Build history of the part. All positions in model axes, mm. A direction names the side the tool comes from. Round coordinates to 2 decimals unless told otherwise and drop trailing zeros. Loops run counter-clockwise (first coordinate to the right, second up) from the corner with the lowest first, then second, coordinate; pieces in that order, holes last. Notation, with made-up numbers: (39, -12.5) -> (86, -12.5) arc R14 cw to (86, 5.5) -> close; hole circle Ø2 at (1.25, 70). An arc over 180 degrees is marked (long way). Put each result on its own line as item: value. Start each with the question number.
Item 1: Tool access for faces 4 (the cylindrical face through (-33.345, 0.986, -28.568)), 5 (the cylindrical face through (36.649, 2.991, 26.096)), 6 (the cylindrical face through (-17.3, 3, 25.3)), 7 (the cylindrical face through (-30.1, 2.9, 21)): list every direction of +Z, -Z, +X, -X, +Y, -Y with a clear straight run to the whole face (end or side of a thin tool).
Item 2: Flat gauge pins, fed straight in: pin 1 Ø1.5 at (x, y) = (-6, 5) entering from -Z; pin 2 Ø3 at (x, y) = (-2.5, 2.5) entering from +Z; pin 3 Ø3 at (y, z) = (3.5, 22.5) entering from +X. Where does each tip first touch, or does it go through?
Item 3: Cut at B-B, the plane x = -1. List the corners of the cut face in (y, z).
Item 4: Pull direction X, two halves, no side cores. Call faces 1 (the flat face through (1, 0, -6)), 2 (the flat face through (29.39, 2.91, 31.54)), 3 (the cylindrical face through (-20.796, 2.909, 36.172)): +X half, -X half, draft (parallel to the pull), parting line (faces both ways), or undercut.
Item 5: Cut at A-A, the plane y = 4.7. Count the separate pieces of the cut face and the enclosed holes in it, plus the area to 3 significant figures.
Item 6: Drill centre lines: probe 1 along X at (y, z) = (2.8, -14.5); probe 2 along X at (y, z) = (0.3, 3.5); probe 3 along X at (y, z) = (0.85, -35). Where is each one in solid material? Low to high. Write a range as [from, to].
Item 7: Cut at D-D, the plane z = 15. List the corners of the cut face in (x, y), plus the area to 3 significant figures.
Item 8: Cut at C-C, the plane x = -46.5. List the corners of the cut face in (y, z).
```python
from build123d import *

# Parameters (mm, degrees)
RESSALTO_EXTRUS_O1_DEPTH = 5.9
FILETE1_R                = 8
FILETE2_R                = 3
ESBO_O2_R                = 1.5
CORTE_EXTRUS_O2_DEPTH    = 2
ESBO_O4_R                = 1.5
ESBO_O4_R_2              = 1.9
CORTE_EXTRUS_O3_DEPTH    = 78.327505241


with BuildPart() as part:
    # Esboço1 → Ressalto-extrusão1 (new body)
    with BuildSketch(Plane(origin=(0, 0, 0), x_dir=(1, 0, 0), z_dir=(0, 1, 0))):
        with BuildLine():
            Line((19.75, -23.063762314), (-19.75, -23.063762314))
            Line((-19.75, -23.063762314), (-19.75, -34.413762314))
            ThreePointArc((-19.75, -34.413762314), (-20.823151937, -36.186035619), (-22.890952667, -36.056390395))
            Line((-22.890952667, -36.056390395), (-37, -26.256390395))
            Line((-37, -26.256390395), (-37, -18.556390395))
            ThreePointArc((-37, -18.556390395), (-37.501443682, -9.224461006), (-39, 0))
            Line((-39, 0), (-60, 39.799497484))
            ThreePointArc((-60, 39.799497484), (-59.849748252, 45.058892271), (-55.268281966, 47.646164151))
            Line((-55.268281966, 47.646164151), (-49.818281966, 47.646164151))
            Line((-49.818281966, 47.646164151), (-16.15, 25.136237686))
            Line((-16.15, 25.136237686), (16.15, 25.136237686))
            Line((16.15, 25.136237686), (49.818281966, 47.646164151))
            Line((49.818281966, 47.646164151), (55.268281966, 47.646164151))
            ThreePointArc((55.268281966, 47.646164151), (59.849748252, 45.058892271), (60, 39.799497484))
            Line((60, 39.799497484), (39, 0))
            ThreePointArc((39, 0), (37.501443682, -9.224461006), (37, -18.556390395))
            Line((37, -18.556390395), (37, -26.256390395))
            Line((37, -26.256390395), (22.890952667, -36.056390395))
            ThreePointArc((22.890952667, -36.056390395), (20.823151937, -36.186035619), (19.75, -34.413762314))
            Line((19.75, -34.413762314), (19.75, -23.063762314))
        make_face()
    extrude(amount=RESSALTO_EXTRUS_O1_DEPTH)

    # Filete1
    filete1_edges = [part.edges().sort_by_distance(p)[0] for p in [
        (19.75, 2.95, 23.063762314),
        (-19.75, 2.95, 23.063762314),
    ]]
    fillet(filete1_edges, radius=FILETE1_R)

    # Filete2
    filete2_edges = [part.edges().sort_by_distance(p)[0] for p in [
        (-37, 2.95, 26.256390395),
        (-39, 2.95, 0),
        (-49.818281966, 2.95, -47.646164151),
        (-16.15, 2.95, -25.136237686),
        (16.15, 2.95, -25.136237686),
        (49.818281966, 2.95, -47.646164151),
        (39, 2.95, 0),
        (37, 2.95, 26.256390395),
    ]]
    fillet(filete2_edges, radius=FILETE2_R)

    # Esboço2 → Corte-extrusão2 (cut)
    # profile 1 of 2: a face of its own
    with BuildSketch(Plane.XZ):
        with BuildLine():
            Line((-52.946039299, -45.974436707), (-34.750912081, -34.487114845))
            ThreePointArc((-34.750912081, -34.487114845), (-33.394882191, -28.486599622), (-39.395397414, -27.130569732))
            Line((-39.395397414, -27.130569732), (-57.590524632, -38.617891595))
            ThreePointArc((-57.590524632, -38.617891595), (-58.946554522, -44.618406817), (-52.946039299, -45.974436707))
        make_face()
        with Locations(Location((-55.268281966, -42.146164151, 0), (0, 0, 270))):
            Circle(ESBO_O2_R, mode=Mode.SUBTRACT)
    # profile 2 of 2: a face of its own
    with BuildSketch(Plane.XZ):
        with BuildLine():
            Line((39.395397414, -27.130569732), (57.590524632, -38.617891595))
            ThreePointArc((57.590524632, -38.617891595), (58.946554522, -44.618406817), (52.946039299, -45.974436707))
            Line((52.946039299, -45.974436707), (34.750912081, -34.487114845))
            ThreePointArc((34.750912081, -34.487114845), (33.394882191, -28.486599622), (39.395397414, -27.130569732))
        make_face()
        with Locations(Location((55.268281966, -42.146164151, 0), (0, 0, 90))):
            Circle(ESBO_O2_R, mode=Mode.SUBTRACT)
    extrude(amount=-CORTE_EXTRUS_O2_DEPTH, mode=Mode.SUBTRACT)

    # Esboço4 → Corte-extrusão3 (cut, through all)
    with BuildSketch(Plane.XZ):
        with Locations(Location((-55.268281966, -42.146164151, 0), (0, 0, 270))):
            Circle(ESBO_O4_R)
        with Locations(Location((55.268281966, -42.146164151, 0), (0, 0, 90))):
            Circle(ESBO_O4_R)
        with Locations(Location((-22.5, -14.736237686, 0), (0, 0, 270))):
            Circle(ESBO_O4_R)
        with Locations(Location((-22.5, -9.736237686, 0), (0, 0, 270))):
            Circle(ESBO_O4_R_2)
        with Locations(Location((-16, 3.863762314, 0), (0, 0, 270))):
            Circle(ESBO_O4_R)
        with Locations(Location((-16, 18.863762314, 0), (0, 0, 270))):
            Circle(ESBO_O4_R)
        with Locations(Location((16, 18.863762314, 0), (0, 0, 90))):
            Circle(ESBO_O4_R)
        with Locations(Location((16, 3.863762314, 0), (0, 0, 90))):
            Circle(ESBO_O4_R)
        with Locations(Location((22.5, -9.736237686, 0), (0, 0, 90))):
            Circle(ESBO_O4_R_2)
        with Locations(Location((22.5, -14.736237686, 0), (0, 0, 90))):
            Circle(ESBO_O4_R)
        with BuildLine():
            ThreePointArc((-32.465664485, 19.788762314), (-31.6, 17.063762314), (-30.734335515, 19.788762314))
            ThreePointArc((-30.734335515, 19.788762314), (-30.1, 21.013762314), (-30.734335515, 22.238762314))
            ThreePointArc((-30.734335515, 22.238762314), (-31.6, 24.963762314), (-32.465664485, 22.238762314))
            ThreePointArc((-32.465664485, 22.238762314), (-33.1, 21.013762314), (-32.465664485, 19.788762314))
        make_face()
        with BuildLine():
            ThreePointArc((-27.965664485, 19.788762314), (-27.1, 17.063762314), (-26.234335515, 19.788762314))
            ThreePointArc((-26.234335515, 19.788762314), (-25.6, 21.013762314), (-26.234335515, 22.238762314))
            ThreePointArc((-26.234335515, 22.238762314), (-27.1, 24.963762314), (-27.965664485, 22.238762314))
            ThreePointArc((-27.965664485, 22.238762314), (-28.6, 21.013762314), (-27.965664485, 19.788762314))
        make_face()
        with BuildLine():
            ThreePointArc((26.234335515, 19.788762314), (25.6, 21.013762314), (26.234335515, 22.238762314))
            ThreePointArc((26.234335515, 22.238762314), (27.1, 24.963762314), (27.965664485, 22.238762314))
            ThreePointArc((27.965664485, 22.238762314), (28.6, 21.013762314), (27.965664485, 19.788762314))
            ThreePointArc((27.965664485, 19.788762314), (27.1, 17.063762314), (26.234335515, 19.788762314))
        make_face()
        with BuildLine():
            ThreePointArc((30.734335515, 19.788762314), (30.1, 21.013762314), (30.734335515, 22.238762314))
            ThreePointArc((30.734335515, 22.238762314), (31.6, 24.963762314), (32.465664485, 22.238762314))
            ThreePointArc((32.465664485, 22.238762314), (33.1, 21.013762314), (32.465664485, 19.788762314))
            ThreePointArc((32.465664485, 19.788762314), (31.6, 17.063762314), (30.734335515, 19.788762314))
        make_face()
    extrude(amount=-CORTE_EXTRUS_O3_DEPTH, mode=Mode.SUBTRACT)


solid = part.part
```
Reply:
1. face 4: -Y
1. face 5: +Z, +X, +Y, -Y
1. face 6: +Z, +Y, -Y
1. face 7: +Y, -Y
2. pin 1: stops at z = -25.14
2. pin 2: stops at z = 23.06
2. pin 3: stops at x = 37
3. outline: (0, -25.14) -> (5.9, -25.14) -> (5.9, 23.06) -> (0, 23.06) -> close
4. face 1: draft
4. face 2: +X half
4. face 3: undercut
5. separate pieces: 1
5. enclosed holes: 14
5. area: 5,300 mm^2
6. probe 1: x = [-46.65, -23.98], [-21.02, 21.02], [23.98, 46.65]
6. probe 2: x = [-38.31, -17.46], [-14.54, 14.54], [17.46, 38.31]
6. probe 3: x = [-57.47, -51.86], [-35.56, -30.9], [30.9, 35.56], [51.86, 57.47]
7. outline: (-37.07, 0) -> (37.07, 0) -> (37.07, 5.9) -> (-37.07, 5.9) -> close
7. area: 437 mm^2
8. outline: (0, -45.43) -> (5.9, -45.43) -> (5.9, -14.21) -> (0, -14.21) -> (0, -31.62) -> (2, -31.62) -> (2, -41.9) -> (0, -41.9) -> close
